Part model, mm, in its own coordinate system. Face numbers are marked on the shaded views. A direction names the side the tool comes from. Round coordinates to 2 decimals unless told otherwise and drop trailing zeros. Loops run counter-clockwise (first coordinate to the right, second up) from the corner with the lowest first, then second, coordinate; pieces in that order, holes last. Notation, with made-up numbers: M 53.25,13.5 L 94.25,13.5 A25 ccw 94.25,34.5 Z; hole C 20.25,-19 d9. An arc over 180 degrees is marked long. Put each result on its own line as item: value. Start each with the question number.
```python
from build123d import *

# Parameters (mm, degrees)
BOSS_EXTRUDE1_DEPTH                                = 4.365625
SKETCH3_W                                          = 44.45
SKETCH3_H                                          = 8.73125
FILLET3_R                                          = 9.525
FILLET2_R                                          = 0.79375
CSK_FOR_10_FLAT_HEAD_MACHINE_SCREW_100_D           = 5.1054
CSK_FOR_10_FLAT_HEAD_MACHINE_SCREW_100_CSINK_D     = 9.779
CSK_FOR_10_FLAT_HEAD_MACHINE_SCREW_100_CSINK_ANGLE = 100
CSK_FOR_10_FLAT_HEAD_MACHINE_SCREW_2_D             = 5.1054
CSK_FOR_10_FLAT_HEAD_MACHINE_SCREW_2_CSINK_D       = 9.779
CSK_FOR_10_FLAT_HEAD_MACHINE_SCREW_2_CSINK_ANGLE   = 100
SKETCH6_R                                          = 1.15
CUT_EXTRUDE1_DEPTH                                 = 90.9706
SKETCH7_R                                          = 1.905
CUT_EXTRUDE2_DEPTH                                 = 6.35
CIRPATTERN1_COUNT                                  = 4


with BuildPart() as part:
    # Sketch1 → Boss-Extrude1 (new body, symmetric)
    with BuildSketch(Plane(origin=(0, 0, 0), x_dir=(1, 0, 0), z_dir=(0, 1, 0))):
        Polygon((-22.225, 9.525), (-22.225, -25.4), (0, -25.4), (0, -12.7), (0, 14.2875), (-17.4625, 14.2875), (-22.225, 14.2875), align=None)
    boss_extrude1 = extrude(amount=BOSS_EXTRUDE1_DEPTH, both=True)

    # Mirror1: Boss-Extrude1 across plane
    add(boss_extrude1.mirror(Plane(origin=(0, 4.365625, 25.4), x_dir=(0, 0, 1), z_dir=(-1, 0, 0))))

    # Sweep1: sweep along a path in Sketch2
    with BuildLine(Plane(origin=(0, 0, 0), x_dir=(0, 0, -1), z_dir=(1, 0, 0))) as sweep1_path:
        Line((-66.368982, -83.523553), (-72.942986, -58.989037))
        ThreePointArc((-72.942986, -58.989037), (-72.98896, -55.884372), (-71.5574, -53.12907))
        Line((-71.5574, -53.12907), (-30.148043, -6.499159))
        ThreePointArc((-30.148043, -6.499159), (-28.002685, -4.923516), (-25.4, -4.365625))
    # Sketch3 → Sweep1 (sweep)
    with BuildSketch(Plane.XY.offset(25.4)):
        Rectangle(SKETCH3_W, SKETCH3_H)
    sweep(path=sweep1_path.line)

    # Fillet3
    fillet3_edges = [part.edges().sort_by_distance(p)[0] for p in [
        (-22.225, -84.65346, 70.585852),
        (22.225, -84.65346, 70.585852),
    ]]
    fillet(fillet3_edges, radius=FILLET3_R)

    # Fillet2
    fillet2_edges = [part.edges().sort_by_distance(p)[0] for p in [
        (-22.225, 0, -14.2875),
        (-22.225, 4.365625, 5.55625),
        (22.225, 4.365625, 5.55625),
        (22.225, 0, -14.2875),
        (22.225, -4.365625, 5.55625),
        (-22.225, -4.923516, 28.002685),
        (22.225, -4.923516, 28.002685),
        (22.225, 3.040634, 31.581378),
        (-22.225, 3.040634, 31.581378),
        (-22.225, -29.814115, 50.852722),
        (22.225, -29.814115, 50.852722),
        (22.225, -24.016474, 57.381282),
        (-22.225, -24.016474, 57.381282),
        (-22.225, -55.884372, 72.98896),
        (22.225, -55.884372, 72.98896),
        (22.225, -53.875272, 81.485915),
        (-22.225, -53.875272, 81.485915),
        (-22.225, -66.656073, 70.88861),
        (22.225, -66.656073, 70.88861),
        (22.225, -68.915887, 79.32235),
        (-22.225, -68.915887, 79.32235),
        (0, -83.523553, 66.368982),
        (0, -85.783366, 74.802722),
        (-19.435192, -83.088619, 75.524777),
        (19.435192, -83.088619, 75.524777),
        (-19.435192, -80.828805, 67.091038),
        (19.435192, -80.828805, 67.091038),
        (-22.225, -4.365625, 5.55625),
        (0, 4.365625, -14.2875),
        (0, -4.365625, -14.2875),
    ]]
    fillet(fillet2_edges, radius=FILLET2_R)

    # CSK for #10 Flat Head Machine Screw (100)1 (through all)
    with Locations(Plane(origin=(-12.7, -74.323109, 68.834233), x_dir=(0, -0.965926, -0.258819), z_dir=(0, 0.258819, -0.965926))):
        with Locations((0, 0)):
            CounterSinkHole(CSK_FOR_10_FLAT_HEAD_MACHINE_SCREW_100_D / 2, CSK_FOR_10_FLAT_HEAD_MACHINE_SCREW_100_CSINK_D / 2, counter_sink_angle=CSK_FOR_10_FLAT_HEAD_MACHINE_SCREW_100_CSINK_ANGLE)

    # CSK for _10 Flat Head Machine Screw  2 (through all)
    with Locations(Plane(origin=(12.7, -74.323109, 68.834233), x_dir=(0, -0.965926, -0.258819), z_dir=(0, 0.258819, -0.965926))):
        with Locations((0, 0)):
            CounterSinkHole(CSK_FOR_10_FLAT_HEAD_MACHINE_SCREW_2_D / 2, CSK_FOR_10_FLAT_HEAD_MACHINE_SCREW_2_CSINK_D / 2, counter_sink_angle=CSK_FOR_10_FLAT_HEAD_MACHINE_SCREW_2_CSINK_ANGLE)

    # Sketch6 → Cut-Extrude1 (cut, through all)
    with BuildSketch(Plane(origin=(0, 4.365625, 0), x_dir=(1, 0, 0), z_dir=(0, 1, 0))):
        with Locations((-11.1125, 11.1125)):
            Circle(SKETCH6_R)
    cut_extrude1 = extrude(amount=-CUT_EXTRUDE1_DEPTH, mode=Mode.SUBTRACT)

    # Sketch7 → Cut-Extrude2 (cut)
    with BuildSketch(Plane.XZ.offset(4.365625)):
        with Locations((-11.1125, -11.1125)):
            Circle(SKETCH7_R)
    cut_extrude2 = extrude(amount=-CUT_EXTRUDE2_DEPTH, mode=Mode.SUBTRACT)

    # CirPattern1: Cut-Extrude1, Cut-Extrude2 ×4 about axis
    cirpattern1_axis = Axis((0, 0, 0), (0, 1, 0))
    for i in range(1, CIRPATTERN1_COUNT):
        add(cut_extrude1.rotate(cirpattern1_axis, i * 360 / CIRPATTERN1_COUNT), mode=Mode.SUBTRACT)
        add(cut_extrude2.rotate(cirpattern1_axis, i * 360 / CIRPATTERN1_COUNT), mode=Mode.SUBTRACT)


solid = part.part
```
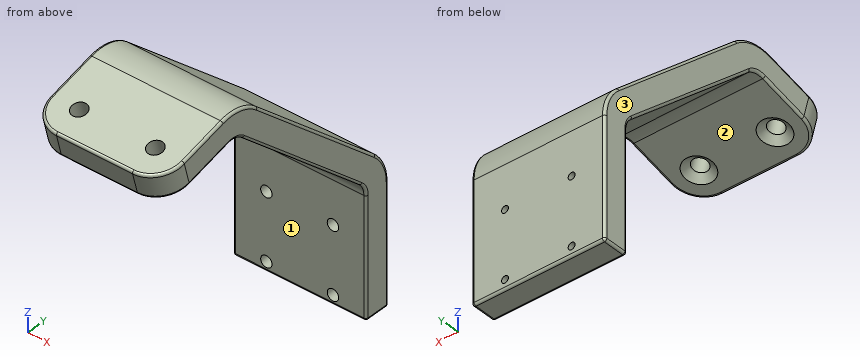
1. Cut at B-B, the plane z = 24. Give the cut face in (x, y) (1 decimal).
2. Wall check: L1, parallel to Z at x = 10, y = -1; L2, parallel to Y at x = -1, z = -8; L3, parallel to Z at x = 6, y = -54.5. Give the ranges that are in metal, low to high.
3. Drop flat-ended pins along their axis: pin 1 (8 mm diameter, centred on x = 12.5, y = -24, fed in from +Z); pin 2 (8 mm diameter, centred on x = -12.5, y = -60, fed in from -Z); pin 3 (4 mm diameter, centred on x = -10, z = -10.5, fed in from -Y); pin 4 (3.5 mm diameter, centred on x = 11.11, z = -11.11, fed in from +Y). Give the stop position or say it passes through.
4. Which spindle directions (+Z, -Z, +X, -X, +Y, -Y) get a long thin tool onto all of the face, cutting with end or side? Do the marked faces 1, 2 and 3. Say none if no direction does.
5. Cut at A-A, the plane x = -2. Give the cut face in (y, z), and give its area (3 significant figures).
Results list:
1. outline: M -22.2,-3.6 A0.8 ccw -21.4,-4.4 L 21.4,-4.4 A0.8 ccw 22.2,-3.6 L 22.2,3.6 A0.8 ccw 21.4,4.4 L -21.4,4.4 A0.8 ccw -22.2,3.6 Z
2. L1: z = -14.29 to -12.66, -9.57 to 9.57, 12.66 to 36.94
2. L2: y = -4.37 to 4.37
2. L3: z = 72.49 to 81.62
3. pin 1: stops at z = 60.92
3. pin 2: stops at z = 71.6
3. pin 3: stops at y = -4.37
3. pin 4: stops at y = 4.37
4. face 1: -Z, +X, -X, -Y
4. face 2: -Z, +X, -X
4. face 3: +Z, -Z, -X, +Y, -Y
5. outline: M -85.58,74.04 L -83.73,67.14 A0.79 ccw -82.76,66.57 L -58.99,72.94 A6.35 cw -53.13,71.56 L -6.5,30.15 A6.35 cw -4.37,25.4 L -4.37,-13.49 A0.79 ccw -3.57,-14.29 L 3.57,-14.29 A0.79 ccw 4.37,-13.49 L 4.37,25.4 A15.08 ccw -0.7,36.68 L -47.33,78.09 A15.08 ccw -61.25,81.38 L -85.02,75.01 A0.79 ccw Z
5. area: 1,280 mm^2
